from build123d import *

# Parameters (mm, degrees)
SKETCH_1_W          = 130
SKETCH_1_H          = 95
EXTRUDE_1_DEPTH     = 3
SKETCH_3_R          = 1.5
CUT_EXTRUDE_2_DEPTH = 10
SKETCH_4_R          = 1.5
CUT_EXTRUDE_3_DEPTH = 10
SKETCH_5_R          = 14
CUT_EXTRUDE_4_DEPTH = 10
SKETCH_6_R          = 1.25
SKETCH_6_R_2        = 1.145522231
CUT_EXTRUDE_5_DEPTH = 10


with BuildPart() as part:
    # 草图1 → 凸台-拉伸1 (new body)
    with BuildSketch(Plane.XY):
        Rectangle(SKETCH_1_W, SKETCH_1_H)
    extrude(amount=EXTRUDE_1_DEPTH)

    # 草图3 → 切除-拉伸2 (cut)
    with BuildSketch(Plane(origin=(0, 0, 0), x_dir=(-1, 0, 0), z_dir=(0, 0, -1))):
        with Locations((-57.767112616, -26.5)):
            Circle(SKETCH_3_R)
        with Locations((-41.767112616, -26.5)):
            Circle(SKETCH_3_R)
        with Locations((42.232887384, -26.5)):
            Circle(SKETCH_3_R)
        with Locations((58.232887384, -26.5)):
            Circle(SKETCH_3_R)
    extrude(amount=-CUT_EXTRUDE_2_DEPTH, mode=Mode.SUBTRACT)

    # 草图4 → 切除-拉伸3 (cut)
    with BuildSketch(Plane(origin=(0, 0, 0), x_dir=(-1, 0, 0), z_dir=(0, 0, -1))):
        with Locations((-46.767112616, 42.5)):
            Circle(SKETCH_4_R)
        with Locations((-46.767112616, 22.5)):
            Circle(SKETCH_4_R)
        with Locations((47.232887384, 42.5)):
            Circle(SKETCH_4_R)
        with Locations((47.232887384, 22.5)):
            Circle(SKETCH_4_R)
    extrude(amount=-CUT_EXTRUDE_3_DEPTH, mode=Mode.SUBTRACT)

    # 草图5 → 切除-拉伸4 (cut)
    with BuildSketch(Plane(origin=(0, 0, 0), x_dir=(-1, 0, 0), z_dir=(0, 0, -1))):
        with Locations((-3.85, -21.35)):
            Circle(SKETCH_5_R)
        with Locations((43.85, 0.996699625)):
            Circle(SKETCH_5_R)
    extrude(amount=-CUT_EXTRUDE_4_DEPTH, mode=Mode.SUBTRACT)

    # 草图6 → 切除-拉伸5 (cut)
    with BuildSketch(Plane.XY.offset(3)):
        with Locations((-59.35, 16.496699625)):
            Circle(SKETCH_6_R)
        with Locations((-28.35, 16.496699625)):
            Circle(SKETCH_6_R)
        with Locations((-59.35, -14.503300375)):
            Circle(SKETCH_6_R)
        with Locations((-28.35, -14.503300375)):
            Circle(SKETCH_6_R)
        with Locations((-11.65, -5.85)):
            Circle(SKETCH_6_R)
        with Locations((19.35, -5.85)):
            Circle(SKETCH_6_R)
        with Locations((19.35, -36.85)):
            Circle(SKETCH_6_R_2)
        with Locations((-11.65, -36.85)):
            Circle(SKETCH_6_R)
    extrude(amount=-CUT_EXTRUDE_5_DEPTH, mode=Mode.SUBTRACT)


solid = part.part
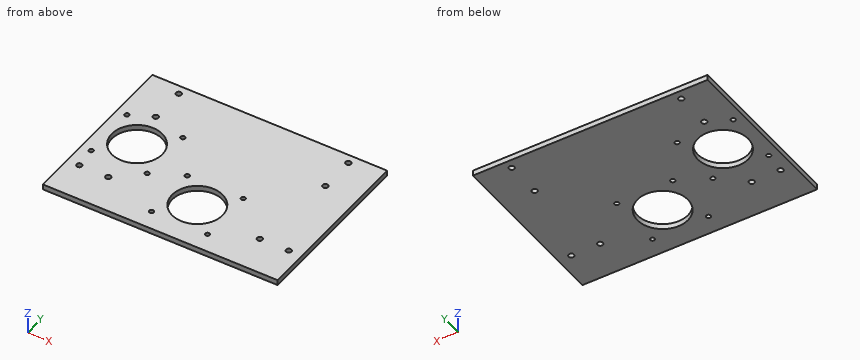
Model file for the job. Use its own axes, mm. Coordinates: 2 decimals unless noted, no trailing zeros. Loops run counter-clockwise (first coordinate to the right, second up) from the corner with the lowest first, then second, coordinate; pieces in that order, holes last. Notation, with made-up numbers: (55, 66.25) -> (73, 66.25) arc R14 cw to (73, 82.25) -> close; hole circle Ø8 at (-33.75, 36.25). An arc over 180 degrees is marked (long way). Use one line per item in the form item = value. Start each with the question number.
(1) Cut at A-A on y = 42.5. Give the cut face in (x, z), and give its area (3 significant figures).
(2) Cut at C-C on x = 0. Give the cut face in (y, z).
(3) Cut at D-D on z = 2.15. Give the number of separate pieces and of enclosed holes in the cut face, and give its area (3 significant figures).
(4) Probe probe 1 along Y at (x, z) = (-59.35, 2.1); probe 2 along Y at (x, z) = (48, 0.5); probe 3 along X at (y, z) = (-20.5, 0.8). List the from-to ranges inside material, lowest first. Write a range as from..to.
(5) Cut at B-B on y = -21.35. Give the cut face in (x, z).
(6) Flat gauge pin, fed straight in: pin 1 (1.8 mm diameter, centred on x = 19.35, y = -36.85, fed in from -Z). Where does the tip first touch, or does it go through?
Values:
q1.outline = (-65, 0) -> (-48.73, 0) -> (-48.73, 3) -> (-65, 3) -> close; (-45.73, 0) -> (45.27, 0) -> (45.27, 3) -> (-45.73, 3) -> close; (48.27, 0) -> (65, 0) -> (65, 3) -> (48.27, 3) -> close
q1.area = 372 mm2
q2.outline = (-47.5, 0) -> (-34.81, 0) -> (-34.81, 3) -> (-47.5, 3) -> close; (-7.89, 0) -> (47.5, 0) -> (47.5, 3) -> (-7.89, 3) -> close
q3.separate_pieces = 1
q3.enclosed_holes = 18
q3.area = 11,000 mm2
q4.probe_1 = -47.5..-27.5, -25.5..-15.75, -13.25..15.25, 17.75..47.5
q4.probe_2 = -47.5..21.65, 23.35..41.65, 43.35..47.5
q4.probe_3 = -65..-10.12, 17.82..65
q5.outline = (-65, 0) -> (-10.15, 0) -> (-10.15, 3) -> (-65, 3) -> close; (17.85, 0) -> (65, 0) -> (65, 3) -> (17.85, 3) -> close
q6.pin_1 = through
